The model under review builds one solid part; all positions refer to its coordinate system, in mm. A direction names the side the tool comes from. Coordinates: 2 decimals unless noted, no trailing zeros. Order: outer loops, then holes, each group sorted by start corner. A loop starts at its lowest first (then second) coordinate and runs counter-clockwise, first axis right, second up. Notation, with made-up numbers: M -30.5,71.25 L 1.5,71.25 A22 cw 1.5,100.25 Z; hole C 73.25,2.5 d11. An arc over 180 degrees is marked long. Answer in a Markdown table with one row per item.
from build123d import *

# Parameters (mm, degrees)
SKETCH_1_R      = 10
EXTRUDE_1_DEPTH = 10
SKETCH_1_3_R    = 37
SKETCH_1_3_R_2  = 12
SKETCH_1_3_R_3  = 7
EXTRUDE_2_DEPTH = 20
EXTRUDE_3_DEPTH = 15


with BuildPart() as part:
    # Sketch 1 → Extrude 1 (new body)
    with BuildSketch(Plane.XY):
        with BuildLine():
            ThreePointArc((33.777631107, 15.102040816), (38.204732973, 9.930851322), (44.732538493, 8))
            Line((44.732538493, 8), (80.358983849, 8))
            ThreePointArc((80.358983849, 8), (86.358983849, 9.607695155), (90.751288694, 14))
            ThreePointArc((90.751288694, 14), (143, 0), (90.751288694, -14))
            ThreePointArc((90.751288694, -14), (86.358983849, -9.607695155), (80.358983849, -8))
            Line((80.358983849, -8), (44.732538493, -8))
            ThreePointArc((44.732538493, -8), (38.204732973, -9.930851322), (33.777631107, -15.102040816))
            ThreePointArc((33.777631107, -15.102040816), (25.981771895, -26.342883843), (14.634400462, -33.982853369))
            ThreePointArc((14.634400462, -33.982853369), (26.793614992, -33.778427283), (35.584428164, -42.181396508))
            ThreePointArc((35.584428164, -42.181396508), (46.651328728, -55.153944971), (63, -60))
            Line((63, -60), (126.630372484, -60))
            ThreePointArc((126.630372484, -60), (142.940084207, -56.940354118), (157.031931827, -48.177480156))
            Line((157.031931827, -48.177480156), (173.401559343, -33.177480156))
            ThreePointArc((173.401559343, -33.177480156), (188, -1.233e-06), (173.401561161, 33.177478491))
            Line((173.401561161, 33.177478491), (157.031931827, 48.177480156))
            ThreePointArc((157.031931827, 48.177480156), (142.940084207, 56.940354118), (126.630372484, 60))
            Line((126.630372484, 60), (115, 60))
            Line((115, 60), (63, 60))
            ThreePointArc((63, 60), (46.651328728, 55.153944971), (35.584428164, 42.181396508))
            ThreePointArc((35.584428164, 42.181396508), (26.793614992, 33.778427283), (14.634400462, 33.982853369))
            ThreePointArc((14.634400462, 33.982853369), (25.981771895, 26.342883843), (33.777631107, 15.102040816))
        make_face()
        with Locations((129.83281573, -45.650712782)):
            Circle(SKETCH_1_R, mode=Mode.SUBTRACT)
        with Locations((76.16718427, -28.21369211)):
            Circle(SKETCH_1_R, mode=Mode.SUBTRACT)
        with Locations((163, 0)):
            Circle(SKETCH_1_R, mode=Mode.SUBTRACT)
        with Locations((76.16718427, 28.21369211)):
            Circle(SKETCH_1_R, mode=Mode.SUBTRACT)
        with Locations((129.83281573, 45.650712782)):
            Circle(SKETCH_1_R, mode=Mode.SUBTRACT)
    extrude(amount=EXTRUDE_1_DEPTH)

    # Sketch 1_3 → Extrude 2 (add)
    with BuildSketch(Plane.XY):
        with Locations(Location((0, 0, 0), (0, 0, 66.701320384))):
            Circle(SKETCH_1_3_R)
        Circle(SKETCH_1_3_R_2, mode=Mode.SUBTRACT)
        with Locations((12, -20.784609691)):
            Circle(SKETCH_1_3_R_3, mode=Mode.SUBTRACT)
        with Locations((12, 20.784609691)):
            Circle(SKETCH_1_3_R_3, mode=Mode.SUBTRACT)
        with Locations((-24, 0)):
            Circle(SKETCH_1_3_R_3, mode=Mode.SUBTRACT)
    extrude(amount=EXTRUDE_2_DEPTH)

    # Sketch 1_4 → Extrude 3 (add)
    with BuildSketch(Plane.XY):
        with BuildLine():
            Line((80.358983849, 8), (44.732538493, 8))
            ThreePointArc((44.732538493, 8), (38.204732973, 9.930851322), (33.777631107, 15.102040816))
            ThreePointArc((33.777631107, 15.102040816), (36.185441485, 7.720998933), (37, 0))
            ThreePointArc((37, 0), (36.185441485, -7.720998933), (33.777631107, -15.102040816))
            ThreePointArc((33.777631107, -15.102040816), (38.204732973, -9.930851322), (44.732538493, -8))
            Line((44.732538493, -8), (80.358983849, -8))
            ThreePointArc((80.358983849, -8), (86.358983849, -9.607695155), (90.751288694, -14))
            ThreePointArc((90.751288694, -14), (143, 0), (90.751288694, 14))
            ThreePointArc((90.751288694, 14), (86.358983849, 9.607695155), (80.358983849, 8))
        make_face()
        with BuildLine():
            Line((98.1817412, 12.575618113), (100.303061543, 14.696938457))
            Line((100.303061543, 14.696938457), (102.424381887, 16.8182588))
            Line((102.424381887, 16.8182588), (108.177048434, 11.065592254))
            ThreePointArc((108.177048434, 11.065592254), (115, 13), (121.822951566, 11.065592254))
            Line((121.822951566, 11.065592254), (127.575618113, 16.8182588))
            Line((127.575618113, 16.8182588), (129.696938457, 14.696938457))
            Line((129.696938457, 14.696938457), (131.8182588, 12.575618113))
            Line((131.8182588, 12.575618113), (126.065592254, 6.822951566))
            ThreePointArc((126.065592254, 6.822951566), (128, 0), (126.065592254, -6.822951566))
            Line((126.065592254, -6.822951566), (131.8182588, -12.575618113))
            Line((131.8182588, -12.575618113), (129.696938457, -14.696938457))
            Line((129.696938457, -14.696938457), (127.575618113, -16.8182588))
            Line((127.575618113, -16.8182588), (121.822951566, -11.065592254))
            ThreePointArc((121.822951566, -11.065592254), (115, -13), (108.177048434, -11.065592254))
            Line((108.177048434, -11.065592254), (102.424381887, -16.8182588))
            Line((102.424381887, -16.8182588), (100.303061543, -14.696938457))
            Line((100.303061543, -14.696938457), (98.1817412, -12.575618113))
            Line((98.1817412, -12.575618113), (103.934407746, -6.822951566))
            ThreePointArc((103.934407746, -6.822951566), (102, 0), (103.934407746, 6.822951566))
            Line((103.934407746, 6.822951566), (98.1817412, 12.575618113))
        make_face(mode=Mode.SUBTRACT)
    extrude(amount=EXTRUDE_3_DEPTH)


solid = part.part
(1) To check wall thickness, follow line 1 (Y direction, x = 114, z = 5.75); line 2 (X direction, y = 4, z = 4.5); line 3 (Y direction, x = 67, z = 8.75). State the ranges of each line that lie inside material, in increasing order. Write a range as [from, to].
Report:
| item | result |
|---|---|
| line 1 | [-60, -12.96], [12.96, 60] |
| line 2 | [-36.78, -29.74], [-18.26, -11.31], [11.31, 102.63], [127.37, 153.83], [172.17, 187.82] |
| line 3 | [-60, -32.21], [-24.22, 24.22], [32.21, 60] |
(2) Machinability: for faces 4 (the cylindrical face through (26.631, -33.716, 4.93)), 5 (the cylindrical face through (115, -13, 7)), 6 (the cylindrical face through (86.283, -9.564, 12.465)), 7 (the cylindrical face through (142.98, -1.03, 12.46)), which of the approach directions +Z, -Z, +X, -X, +Y, -Y give a long, thin tool a straight path to every point of the face, cutting with its end or side? Answer none if there is none.
Report:
| item | result |
|---|---|
| face 4 | +Z, -Z, -Y |
| face 5 | +Z, -Z |
| face 6 | +Z, -Y |
| face 7 | +Z |
(3) Take a section at A-A (y = 0). Write out the cut boundary in (x, z), then the cut area to 3 significant figures.
Report:
| item | result |
|---|---|
| outline | M -37,0 L -31,0 L -31,20 L -37,20 Z; M -17,0 L -12,0 L -12,20 L -17,20 Z; M 12,0 L 102,0 L 102,15 L 37,15 L 37,20 L 12,20 Z; M 128,0 L 153,0 L 153,10 L 143,10 L 143,15 L 128,15 Z; M 173,0 L 188,0 L 188,10 L 173,10 Z |
| area | 2,170 mm^2 |
(4) Take a section at D-D (x = 115). Write out the cut boundary in (y, z).
Report:
| item | result |
|---|---|
| outline | M -60,0 L -13,0 L -13,15 L -28,15 L -28,10 L -60,10 Z; M 13,0 L 60,0 L 60,10 L 28,10 L 28,15 L 13,15 Z |
(5) Insertion check: P1, Ø8, axis at y = -23.5, z = 11, coming from the +X side; P2, Ø1.5, axis at x = 67.5, z = 11.5, coming from the -Y side; P3, Ø17, axis at x = 75.5, y = 2.5, coming from the +Z side. Each pin has a flat end and moves straight along its axis. Give the tip position at first contact, or say it passes through.
Report:
| item | result |
|---|---|
| P1 | x = 183.49 |
| P2 | y = -8 |
| P3 | z = 15 |
(6) Take a section at C-C (y = 30.5). Write out the cut boundary in (x, z), then the cut area to 3 significant figures.
Report:
| item | result |
|---|---|
| outline | M -20.95,0 L 66.43,0 L 66.43,10 L 20.95,10 L 20.95,20 L -20.95,20 Z; M 85.9,0 L 176.09,0 L 176.09,10 L 85.9,10 Z |
| area | 2,190 mm^2 |
(7) Take a section at B-B (x = 0). Write out the cut boundary in (y, z).
Report:
| item | result |
|---|---|
| outline | M -37,0 L -12,0 L -12,20 L -37,20 Z; M 12,0 L 37,0 L 37,20 L 12,20 Z |
(8) The part is to be moulded in two halves that separate along Y. For faces 1 (the cylindrical face through (128, 0, 7)), 2 (the cylindrical face through (-35.599, 10.086, 9.86)), 3 (the cylindrical face through (142.722, -57.024, 4.93)), say which applies: +Y half, -Y half, draft (parallel to the pull), parting line (faces both ways), or undercut.
Report:
| item | result |
|---|---|
| face 1 | undercut |
| face 2 | parting line |
| face 3 | -Y half |
